The model under review builds one solid part; all positions refer to its coordinate system, in mm. A direction names the side the tool comes from. Give positions to 0.01 mm unless a question says otherwise; leave off trailing zeros. Order: outer loops, then holes, each group sorted by start corner. A loop starts at its lowest first (then second) coordinate and runs counter-clockwise, first axis right, second up. Notation, with made-up numbers: M 29,81 L 67,81 A25 ccw 67,99 Z; hole C 86,-32 d3. An arc over 180 degrees is marked long. One line per question, with ' | ' between items. Start each with the question number.
1. For faces 1 (the face through (28, 44, 16)), 2 (the face through (28.376, 44.849, 8.465)), 3 (the face through (29, 45, 21)), list the 3-axis set-ups (+Z, -Z, +X, -X, +Y, -Y) from which the entire face can be reached by the end or side of a thin tool; tool diameter is ignored.
2. We need section D-D on z = 18.5. Write out the cut boundary in (x, y) (3 decimals), then the cut area to 3 significant figures.
3. Wall thickness on L1, parallel to Z at x = 27.55, y = 43.8; L2, parallel to X at y = 45.3, z = 9.5; L3, parallel to X at y = 45.2, z = 19: over which ranges is each line inside the solid? List them lowest first.
4. We need section B-B on x = 29.5. Write out the cut boundary in (y, z) (3 decimals).
5. We need section C-C on z = 15.25. Write out the cut boundary in (x, y), then the cut area to 3 significant figures.
6. We need section A-A on y = 44.8. Write out the cut boundary in (x, z) (3 decimals).
7. Insertion check: P1, Ø1.5, axis at y = 46.5, z = 13, coming from the -X side; P2, Ø1.5, axis at x = 30.5, z = 19.5, coming from the +Y side. Each pin has a flat end and moves straight along its axis. Give the tip position at first contact, or say it passes through.
```python
from build123d import *

# Parameters (mm, degrees)
CYLINDER002_R        = 4.5
CYLINDER002_DEPTH    = 10
CYLINDER003_R        = 2.25
CYLINDER003_DEPTH    = 30
CLONE014_SCALE_SCALE = 0.5


with BuildPart() as cylinder002:
    # Cylinder002 → Cylinder002 (new body)
    with BuildSketch(Plane(origin=(0, 10, 5), x_dir=(1, 0, 0), z_dir=(0, 0, 1))):
        Circle(CYLINDER002_R)
    extrude(amount=CYLINDER002_DEPTH)


with BuildPart() as clone014:
    # Cylinder003 → Cylinder003 (new body)
    with BuildSketch(Plane(origin=(0, 10, -5), x_dir=(1, 0, 0), z_dir=(0, 0, 1))):
        Circle(CYLINDER003_R)
    extrude(amount=CYLINDER003_DEPTH)

    # Fusion002: union Cylinder002
    add(cylinder002.part)


with BuildPart() as clone014_1:
    # Clone014 scale: moved
    add(clone014.part.scale(CLONE014_SCALE_SCALE))


with BuildPart() as clone014_2:
    # Clone014 placement: moved
    add(clone014_1.part.moved(Location((29.5, 39.8, 8.5))))


solid = clone014_2.part
```
Entries:
1) face 1: +Z | face 2: -Z | face 3: +Z, +X, -X, +Y, -Y
2) outline: C 29.5,44.8 d2.25 | area: 3.98 mm^2
3) L1: z = 11 to 16 | L2: x = 28.49 to 30.51 | L3: x = 28.45 to 30.55
4) outline: M 42.55,11 L 43.675,11 L 43.675,6 L 45.925,6 L 45.925,11 L 47.05,11 L 47.05,16 L 45.925,16 L 45.925,21 L 43.675,21 L 43.675,16 L 42.55,16 Z
5) outline: C 29.5,44.8 d4.5 | area: 15.9 mm^2
6) outline: M 27.25,11 L 28.375,11 L 28.375,6 L 30.625,6 L 30.625,11 L 31.75,11 L 31.75,16 L 30.625,16 L 30.625,21 L 28.375,21 L 28.375,16 L 27.25,16 Z
7) P1: stops at x = 27.46 | P2: stops at y = 45.9
